The figure shows three views and two pictorial views of one solid part (mm, origin at its lowest corner). Answer the questions. Give positions to 0.01 mm unless a question says otherwise; leave off trailing zeros. Write each loop counter-clockwise with the first axis right and the second up, starting at its lowest first coordinate (ties: lowest second). Pieces come first, ordered by that corner, then holes. Notation, with made-up numbers: (82.5, 20.5) -> (129.5, 20.5) arc R26 cw to (129.5, 50.5) -> close; hole circle Ø1 at (25.5, 26.25). An arc over 180 degrees is marked (long way). Answer as CSV lines item,"result". Start each with the question number.
1. Given pin 1 (1 mm diameter, centred on y = 17.5, z = 35.5, fed in from +X); pin 2 (8 mm diameter, centred on y = 13.5, z = 47, fed in from -X); pin 3 (1 mm diameter, centred on x = 23.5, y = 13, fed in from +Z), each flat-ended and moving along its own axis, determine where each tip first touches the part or whether it passes through.
2. The part is cut by section A-A, the plane x = 17.5. Determine the outline of the cut face in (y, z).
3. Find the intervals of material crossed by line 1 (Y direction, x = 17.5, z = 25); line 2 (X direction, y = 17, z = 22); line 3 (Z direction, x = 9.5, y = 21.5), in increasing order.
4. The part is cut by section C-C, the plane z = 54. Determine the outline of the cut face in (x, y).
5. For a pull along Z with two mould halves and no side action, classify the marked faces 1, 2 and 3 as pulls with the +Z half, pulls with the -Z half, needs draft (parallel to the pull), parting line crosses it, or undercut.
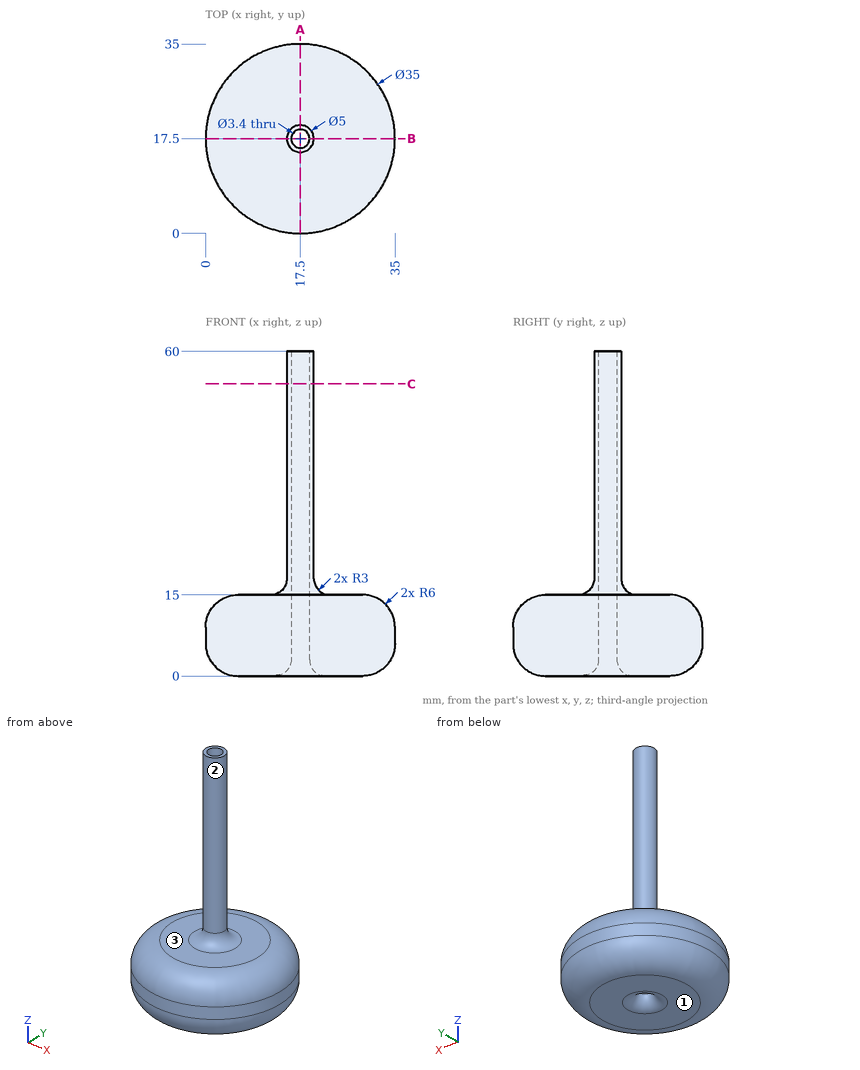
Results found:
1,pin 1,"stops at x = 20"
1,pin 2,"stops at x = 15"
1,pin 3,"stops at z = 15"
2,outline,"(0, 6) arc R6 ccw to (6, 0) -> (12.8, 0) arc R3 ccw to (15.8, 3) -> (15.8, 60) -> (15, 60) -> (15, 18) arc R3 cw to (12, 15) -> (6, 15) arc R6 ccw to (0, 9) -> close; (19.2, 3) arc R3 ccw to (22.2, 0) -> (29, 0) arc R6 ccw to (35, 6) -> (35, 9) arc R6 ccw to (29, 15) -> (23, 15) arc R3 cw to (20, 18) -> (20, 60) -> (19.2, 60) -> close"
3,line 1,"y = 15 to 15.8, 19.2 to 20"
3,line 2,"x = 15.05 to 15.88, 19.12 to 19.95"
3,line 3,"z = 0 to 15"
4,outline,"circle Ø5 at (17.5, 17.5); hole circle Ø3.4 at (17.5, 17.5)"
5,face 1,"pulls with the -Z half"
5,face 2,"needs draft"
5,face 3,"pulls with the +Z half"
